from build123d import *

# Parameters (mm, degrees)
SKETCH3_W                       = 812.8
SKETCH3_H                       = 457.2
BOSS_EXTRUDE3_DEPTH             = 50.8
SKETCH7_W                       = 762
SKETCH7_H                       = 406.4
CUT_EXTRUDE1_DEPTH              = 25.4
SKETCH8_W                       = 355.6
SKETCH8_H                       = 114.3
BOSS_EXTRUDE7_DEPTH             = 25.4
SKETCH23_W                      = 431.8
SKETCH23_H                      = 7.62
CUT_EXTRUDE11_DEPTH             = 5.08
SKETCH24_W                      = 762
SKETCH24_H                      = 7.62
CUT_EXTRUDE12_DEPTH             = 81.026
SKETCH26_W                      = 208.28
SKETCH26_H                      = 7.62
CUT_EXTRUDE13_DEPTH             = 5.08
SKETCH28_W                      = 119.38
SKETCH28_H                      = 7.62
CUT_EXTRUDE14_DEPTH             = 5.08
SKETCH30_W                      = 293.37
SKETCH30_H                      = 77.47
CUT_EXTRUDE16_DEPTH             = 12.7
CUT_EXTRUDE19_REACH             = 520.216
SKETCH32_W                      = 165.1
SKETCH32_H                      = 13.97
CUT_EXTRUDE19_DIRECTION_2_DEPTH = 44.45
FILLET1_R                       = 25.4


with BuildPart() as part:
    # Sketch3 → Boss-Extrude3 (new body)
    with BuildSketch(Plane(origin=(0, 0, 0), x_dir=(1, 0, 0), z_dir=(0, 1, 0))):
        Rectangle(SKETCH3_W, SKETCH3_H)
    extrude(amount=BOSS_EXTRUDE3_DEPTH)

    # Sketch7 → Cut-Extrude1 (cut)
    with BuildSketch(Plane(origin=(0, 50.8, 0), x_dir=(1, 0, 0), z_dir=(0, 1, 0))):
        Rectangle(SKETCH7_W, SKETCH7_H)
    extrude(amount=-CUT_EXTRUDE1_DEPTH, mode=Mode.SUBTRACT)

    # Sketch8 → Boss-Extrude7 (add)
    with BuildSketch(Plane(origin=(0, 25.4, 0), x_dir=(1, 0, 0), z_dir=(0, 1, 0))):
        with Locations((0, -146.05)):
            Rectangle(SKETCH8_W, SKETCH8_H)
    extrude(amount=BOSS_EXTRUDE7_DEPTH)

    # Sketch23 → Cut-Extrude11 (cut)
    with BuildSketch(Plane(origin=(-381, 0, 0), x_dir=(0, 0, -1), z_dir=(1, 0, 0))):
        with Locations((12.7, 43.18)):
            Rectangle(SKETCH23_W, SKETCH23_H)
    cut_extrude11 = extrude(amount=-CUT_EXTRUDE11_DEPTH, mode=Mode.SUBTRACT)

    # Mirror3: Cut-Extrude11 across plane
    add(cut_extrude11.mirror(Plane(origin=(0, 0, 0), x_dir=(0, 0, 1), z_dir=(1, 0, 0))), mode=Mode.SUBTRACT)

    # Sketch24 → Cut-Extrude12 (cut)
    with BuildSketch(Plane(origin=(0, 0, -228.6), x_dir=(-1, 0, 0), z_dir=(0, 0, -1))):
        with Locations((0, 43.18)):
            Rectangle(SKETCH24_W, SKETCH24_H)
    extrude(amount=-CUT_EXTRUDE12_DEPTH, mode=Mode.SUBTRACT)

    # Sketch26 → Cut-Extrude13 (cut)
    with BuildSketch(Plane(origin=(0, 0, 203.2), x_dir=(-1, 0, 0), z_dir=(0, 0, -1))):
        with Locations((-281.94, 43.18)):
            Rectangle(SKETCH26_W, SKETCH26_H)
    cut_extrude13 = extrude(amount=-CUT_EXTRUDE13_DEPTH, mode=Mode.SUBTRACT)

    # Mirror4: Cut-Extrude13 across plane
    add(cut_extrude13.mirror(Plane(origin=(0, 0, 0), x_dir=(0, 0, 1), z_dir=(1, 0, 0))), mode=Mode.SUBTRACT)

    # Sketch28 → Cut-Extrude14 (cut)
    with BuildSketch(Plane(origin=(177.8, 0, 0), x_dir=(0, 0, -1), z_dir=(1, 0, 0))):
        with Locations((-148.59, 43.18)):
            Rectangle(SKETCH28_W, SKETCH28_H)
    cut_extrude14 = extrude(amount=-CUT_EXTRUDE14_DEPTH, mode=Mode.SUBTRACT)

    # Mirror5: Cut-Extrude14 across plane
    add(cut_extrude14.mirror(Plane(origin=(0, 0, 0), x_dir=(0, 0, 1), z_dir=(1, 0, 0))), mode=Mode.SUBTRACT)

    # Sketch30 → Cut-Extrude16 (cut)
    with BuildSketch(Plane(origin=(0, 50.8, 0), x_dir=(1, 0, 0), z_dir=(0, 1, 0))):
        with Locations((0, -146.05)):
            Rectangle(SKETCH30_W, SKETCH30_H)
    extrude(amount=-CUT_EXTRUDE16_DEPTH, mode=Mode.SUBTRACT)

    # Cut-Extrude19: up to this face of the body (flat: up to its plane)
    cut_extrude19_end = Plane(part.part.faces().sort_by_distance((0, 44.45, 184.785))[0])
    # Sketch32 → Cut-Extrude19 (cut, up to the picked face)
    with BuildSketch(Plane(origin=(0, 0, 88.9), x_dir=(-1, 0, 0), z_dir=(0, 0, -1)), mode=Mode.PRIVATE) as cut_extrude19_sk1:
        with Locations((0, 32.385)):
            Rectangle(SKETCH32_W, SKETCH32_H)
    cut_extrude19_tool1 = split(extrude(cut_extrude19_sk1.sketch, amount=-CUT_EXTRUDE19_REACH, mode=Mode.PRIVATE), bisect_by=cut_extrude19_end, keep=Keep.BOTH, mode=Mode.PRIVATE)
    add(cut_extrude19_tool1.solids().sort_by(Axis((0, 32.385, 88.9), (0, 0, 1)))[0], mode=Mode.SUBTRACT)

    # Sketch32 → Cut-Extrude19 direction 2 (cut)
    with BuildSketch(Plane(origin=(0, 0, 88.9), x_dir=(-1, 0, 0), z_dir=(0, 0, -1))):
        with Locations((0, 32.385)):
            Rectangle(SKETCH32_W, SKETCH32_H)
    extrude(amount=CUT_EXTRUDE19_DIRECTION_2_DEPTH, mode=Mode.SUBTRACT)

    # Fillet1
    # the kernel refuses this fillet: 25.4 mm, written as the material it takes off along each edge
    with BuildSketch(Plane(origin=(-406.4, -63.5, -228.6), x_dir=(1, 0, 0), z_dir=(0, 1, 0)), Plane(origin=(-406.4, -63.5, 228.6), x_dir=(0, 0, -1), z_dir=(0, 1, 0))) as fillet1_piece_1:
        with BuildLine():
            CenterArc((FILLET1_R, -FILLET1_R), FILLET1_R, 90, 90)
            Line((0, -FILLET1_R), (0, 0))
            Line((0, 0), (FILLET1_R, 0))
        make_face()
    extrude(amount=177.8, mode=Mode.SUBTRACT)
    with BuildSketch(Plane(origin=(406.4, -63.5, -228.6), x_dir=(-1, 0, 0), z_dir=(0, 1, 0)), Plane(origin=(406.4, -63.5, 228.6), x_dir=(0, 0, -1), z_dir=(0, 1, 0))) as fillet1_piece_2:
        with BuildLine():
            CenterArc((FILLET1_R, FILLET1_R), FILLET1_R, 180, 90)
            Line((0, FILLET1_R), (0, 0))
            Line((0, 0), (FILLET1_R, 0))
        make_face()
    extrude(amount=177.8, mode=Mode.SUBTRACT)


solid = part.part
Geometry: final body of the model. Coordinates: model frame, mm. A direction names the side the tool comes from. Coordinates: 2 decimals unless noted, no trailing zeros. Loops run counter-clockwise (first coordinate to the right, second up) from the corner with the lowest first, then second, coordinate; pieces in that order, holes last. Notation, with made-up numbers: (-33, -21) - (-27, -21) arc R35 ccw to (-27, 18) - close; hole circle Ø1 at (30.25, 11). An arc over 180 degrees is marked (long way). One line per question, with ' | ' between items. Start each with the question number.
(1) Draft query along Z for faces 4 (the flat face through (-2, 50.8, 101)), 5 (the flat face through (-2, 41, 88.9)), 6 (the flat face through (-5, 19, -228.6)), 7 (the cylindrical face through (398.76, 25.04, 221.36)). Return one class per face: +Z half, -Z half, draft (parallel to the pull), parting line (faces both ways), or undercut.
(2) First-contact query: pin 1 (1 mm diameter, centred on x = -307.5, z = -92.5, fed in from -Y). Flat tip, straight axial feed; report the tip coordinate or a pass-through.
(3) Cut plane D-D on z = -18. Output: boundary loops of the cut face in (x, y), and give its area (3 significant figures).
(4) Reachability of faces 1 (the flat face through (30, 46.99, -219)), 2 (the flat face through (1, 39.37, 98)), 3 (the flat face through (-2, 41, 184.785)) from +Z, -Z, +X, -X, +Y, -Y: full face, straight path, thin tool, end or side. Return the list, or none.
(5) Ray query, L1, parallel to X at y = 41, z = 153.5 (3 decimals); L2, parallel to Z at x = 165, y = 32; L3, parallel to Z at x = -7, y = 27 (3 decimals). Return the intervals inside material, ascending. Write a range as from..to.
(6) Cut plane A-A on x = 92.5. Output: boundary loops of the cut face in (y, z) (3 decimals), and give its area (3 significant figures).
(7) Cut plane C-C on x = 278.5. Output: boundary loops of the cut face in (y, z).
(8) Cut plane B-B on z = 195. Output: boundary loops of the cut face in (x, y), and give its area (3 significant figures).
Here are the results:
1) face 4: draft | face 5: undercut | face 6: -Z half | face 7: +Z half
2) pin 1: y = 0
3) outline: (-406.4, 0) - (406.4, 0) - (406.4, 50.8) - (381, 50.8) - (381, 46.99) - (386.08, 46.99) - (386.08, 39.37) - (381, 39.37) - (381, 25.4) - (-381, 25.4) - (-381, 39.37) - (-386.08, 39.37) - (-386.08, 46.99) - (-381, 46.99) - (-381, 50.8) - (-406.4, 50.8) - close | area: 21,900 mm²
4) face 1: -Z | face 2: none | face 3: +Y
5) L1: -406.4..-386.08, -172.72..-146.685, 146.685..172.72, 386.08..406.4 | L2: -228.6..-203.2, 88.9..228.6 | L3: -228.6..-203.2, 184.785..228.6
6) outline: (0, -228.6) - (39.37, -228.6) - (39.37, -203.2) - (25.4, -203.2) - (25.4, 88.9) - (50.8, 88.9) - (50.8, 107.315) - (38.1, 107.315) - (38.1, 184.785) - (50.8, 184.785) - (50.8, 228.6) - (0, 228.6) - close; (46.99, -228.6) - (50.8, -228.6) - (50.8, -203.2) - (46.99, -203.2) - close | area: 14,600 mm²
7) outline: (0, -228.6) - (39.37, -228.6) - (39.37, -203.2) - (25.4, -203.2) - (25.4, 203.2) - (39.37, 203.2) - (39.37, 208.28) - (46.99, 208.28) - (46.99, 203.2) - (50.8, 203.2) - (50.8, 228.6) - (0, 228.6) - close; (46.99, -228.6) - (50.8, -228.6) - (50.8, -203.2) - (46.99, -203.2) - close
8) outline: (-406.4, 0) - (406.4, 0) - (406.4, 50.8) - (381, 50.8) - (381, 46.99) - (386.08, 46.99) - (386.08, 39.37) - (381, 39.37) - (381, 25.4) - (177.8, 25.4) - (177.8, 39.37) - (172.72, 39.37) - (172.72, 46.99) - (177.8, 46.99) - (177.8, 50.8) - (-177.8, 50.8) - (-177.8, 46.99) - (-172.72, 46.99) - (-172.72, 39.37) - (-177.8, 39.37) - (-177.8, 25.4) - (-381, 25.4) - (-381, 39.37) - (-386.08, 39.37) - (-386.08, 46.99) - (-381, 46.99) - (-381, 50.8) - (-406.4, 50.8) - close | area: 30,800 mm²
